Can you work these out from the model? Positions are in its coordinate system, mm. A direction names the side the tool comes from. Give positions to 0.01 mm unless a question says otherwise; leave off trailing zeros. Loops run counter-clockwise (first coordinate to the right, second up) from the corner with the lowest first, then second, coordinate; pieces in that order, holes last. Notation, with made-up numbers: (-36.75, -38) -> (13.25, -38) arc R16 ccw to (13.25, -15) -> close; hole circle Ø11 at (86.5, -17). An arc over 180 degrees is marked (long way). Return JSON: item names as keys, results as strings. Group by question number.
Q1. Will these pins go through, and if not, where does the flat tip stop? pin 1 (4 mm diameter, centred on x = -26.5, z = 36, fed in from +Y); pin 2 (3 mm diameter, centred on x = -90.5, y = 1.5, fed in from +Z); pin 3 (4 mm diameter, centred on y = 2, z = 35.5, fed in from -X); pin 4 (6.5 mm diameter, centred on x = 21.5, y = 3, fed in from -Z).
Q2. Thinking about a two-plate mould opening in X: for faces 5 (the flat face through (-99.083, 31, 34)), 6 (the cylindrical face through (-88.32, 22.23, 34.45)), 7 (the flat face through (21, 3, 37.891)), 8 (the cylindrical face through (-9.48, 31.04, 34.45)), which applies, pulls with the +X half, pulls with the -X half, needs draft (parallel to the pull), parting line crosses it, or undercut?
Q3. Which directions (+Z, -Z, +X, -X, +Y, -Y) give clear straight access to the entire face, cutting with the end or side of a thin tool? Please do faces 1 (the flat face through (21, 3, 32.891)), 2 (the flat face through (-94.083, 59, 35)), 3 (the cylindrical face through (20.111, 22.196, 34.447)), 4 (the flat face through (-89, 59, 32.891)).
Q4. Suppose I cut it at D-D, the plane z = 35.75. Count the separate pieces of the cut face and the enclosed holes in it, and give its area (3 significant figures).
Q5. Suppose I cut it at B-B, the plane x = -72. Please give me the cut outline in (y, z).
Q6. I need wall thicknesses on line 1 along X through (y, z) = (29.5, 34); line 2 along Y through (x, z) = (-50, 31.75); line 3 along Y through (x, z) = (-23.5, 36.75). Which ranges of each line are inside material? Lowest first, please. Write a range as [from, to].
Q7. Suppose I cut it at A-A, the plane y = 31. Please give me the cut outline in (x, z).
Q8. Suppose I cut it at C-C, the plane y = 43.5. Please give me the cut outline in (x, z), and give its area (3 significant figures).
```python
from build123d import *

# Parameters (mm, degrees)
SKETCH1_W             = 10
SKETCH1_H             = 5
BOSS_EXTRUDE1_DEPTH   = 6
BOSS_EXTRUDE1_2_DEPTH = 6
SKETCH2_W             = 130
SKETCH2_H             = 8
BOSS_EXTRUDE2_DEPTH   = 50
SKETCH3_W             = 10
SKETCH3_H             = 5
BOSS_EXTRUDE3_DEPTH   = 6
CUT_EXTRUDE1_DEPTH    = 118.155500326


with BuildPart() as part:
    # Sketch1 → Boss-Extrude1 (new body)
    with BuildSketch(Plane(origin=(0, 0, 0), x_dir=(1, 0, 0), z_dir=(0, 1, 0))):
        with Locations((21.089936581, -35.391183382)):
            Rectangle(SKETCH1_W, SKETCH1_H)
    extrude(amount=BOSS_EXTRUDE1_DEPTH)



with BuildPart() as body_2:
    # Sketch1 → Boss-Extrude1 2 (new body)
    with BuildSketch(Plane(origin=(0, 0, 0), x_dir=(1, 0, 0), z_dir=(0, 1, 0))):
        with Locations((-89.082850467, -35.391183382)):
            Rectangle(SKETCH1_W, SKETCH1_H)
    extrude(amount=BOSS_EXTRUDE1_2_DEPTH)


with BuildPart() as part_1:
    add(part.part)

    add(body_2.part)  # Boss-Extrude2 merges body 2
    # Sketch2 → Boss-Extrude2 (add)
    with BuildSketch(Plane(origin=(0, 6, 0), x_dir=(1, 0, 0), z_dir=(0, 1, 0))):
        with Locations((-34.082850467, -34.391183382)):
            Rectangle(SKETCH2_W, SKETCH2_H)
    extrude(amount=BOSS_EXTRUDE2_DEPTH)

    # Sketch3 → Boss-Extrude3 (add)
    with BuildSketch(Plane(origin=(0, 56, 0), x_dir=(1, 0, 0), z_dir=(0, 1, 0))):
        with Locations((-89.082850467, -35.391183382)):
            Rectangle(SKETCH3_W, SKETCH3_H)
        with Locations((21.089936581, -35.391183382)):
            Rectangle(SKETCH3_W, SKETCH3_H)
    extrude(amount=BOSS_EXTRUDE3_DEPTH)

    # Sketch4 → Cut-Extrude1 (cut, through all)
    with BuildSketch(Plane.XY.offset(38.391183382)):
        with BuildLine():
            Line((-13.020277053, 46), (-55.145423882, 46))
            ThreePointArc((-55.145423882, 46), (-57.127727502, 44.265466302), (-55.671658693, 42.070472358))
            Line((-55.671658693, 42.070472358), (-34.609085279, 36.326134154))
            ThreePointArc((-34.609085279, 36.326134154), (-34.082850467, 36.255661796), (-33.556615656, 36.326134154))
            Line((-33.556615656, 36.326134154), (-12.494042241, 42.070472358))
            ThreePointArc((-12.494042241, 42.070472358), (-11.037973433, 44.265466302), (-13.020277053, 46))
        make_face()
        with BuildLine():
            Line((-89.082850467, 38.198883658), (-89.082850467, 23.801116342))
            ThreePointArc((-89.082850467, 23.801116342), (-88.296837777, 22.211702987), (-86.556615656, 21.871588699))
            Line((-86.556615656, 21.871588699), (-60.160708908, 29.070472358))
            ThreePointArc((-60.160708908, 29.070472358), (-58.68694372, 31), (-60.160708908, 32.929527642))
            Line((-60.160708908, 32.929527642), (-86.556615656, 40.128411301))
            ThreePointArc((-86.556615656, 40.128411301), (-88.296837777, 39.788297013), (-89.082850467, 38.198883658))
        make_face()
        with BuildLine():
            Line((-55.145423882, 16), (-13.020277053, 16))
            ThreePointArc((-13.020277053, 16), (-11.037973433, 17.734533698), (-12.494042241, 19.929527642))
            Line((-12.494042241, 19.929527642), (-33.556615656, 25.673865846))
            ThreePointArc((-33.556615656, 25.673865846), (-34.082850467, 25.744338204), (-34.609085279, 25.673865846))
            Line((-34.609085279, 25.673865846), (-55.671658693, 19.929527642))
            ThreePointArc((-55.671658693, 19.929527642), (-57.127727502, 17.734533698), (-55.145423882, 16))
        make_face()
        with BuildLine():
            Line((20.917149533, 23.801116342), (20.917149533, 38.198883658))
            ThreePointArc((20.917149533, 38.198883658), (20.131136843, 39.788297013), (18.390914721, 40.128411301))
            Line((18.390914721, 40.128411301), (-8.004992027, 32.929527642))
            ThreePointArc((-8.004992027, 32.929527642), (-9.478757215, 31), (-8.004992027, 29.070472358))
            Line((-8.004992027, 29.070472358), (18.390914721, 21.871588699))
            ThreePointArc((18.390914721, 21.871588699), (20.131136843, 22.211702987), (20.917149533, 23.801116342))
        make_face()
    extrude(amount=-CUT_EXTRUDE1_DEPTH, mode=Mode.SUBTRACT)


solid = part_1.part
```
Ans:
{
 "1": {"pin 1": "stops at y = 56", "pin 2": "stops at z = 37.89", "pin 3": "stops at x = -94.08", "pin 4": "stops at z = 30.39"},
 "2": {"face 5": "pulls with the -X half", "face 6": "undercut", "face 7": "needs draft", "face 8": "undercut"},
 "3": {"face 1": "-Z, +X, -X, -Y", "face 2": "+Z, -Z, -X, +Y", "face 3": "+Z, -Z", "face 4": "-Z, +X, -X, +Y"},
 "4": {"separate pieces": "1", "enclosed holes": "4", "area": "5,450 mm^2"},
 "5": {"outline": "(6, 30.39) -> (25.84, 30.39) -> (25.84, 38.39) -> (6, 38.39) -> close; (36.16, 30.39) -> (56, 30.39) -> (56, 38.39) -> (36.16, 38.39) -> close"},
 "6": {"line 1": "x = [-99.08, -89.08], [-59.36, -8.8], [20.92, 30.92]", "line 2": "y = [6, 16], [21.48, 40.52], [46, 56]", "line 3": "y = [6, 16], [22.93, 39.07], [46, 56]"},
 "7": {"outline": "(-99.08, 30.39) -> (-89.08, 30.39) -> (-89.08, 38.39) -> (-99.08, 38.39) -> close; (-58.69, 30.39) -> (-9.48, 30.39) -> (-9.48, 38.39) -> (-58.69, 38.39) -> close; (20.92, 30.39) -> (30.92, 30.39) -> (30.92, 38.39) -> (20.92, 38.39) -> close"},
 "8": {"outline": "(-99.08, 30.39) -> (-57.08, 30.39) -> (-57.08, 38.39) -> (-99.08, 38.39) -> close; (-11.08, 30.39) -> (30.92, 30.39) -> (30.92, 38.39) -> (-11.08, 38.39) -> close", "area": "672 mm^2"}
}
